The drawing under review shows one solid part. Ordinate dimensions are in mm from its lowest x, y, z. A direction names the side the tool comes from. Coordinates: 2 decimals unless noted, no trailing zeros. Write each loop counter-clockwise with the first axis right and the second up, starting at its lowest first coordinate (ties: lowest second). Pieces come first, ordered by that corner, then holes.
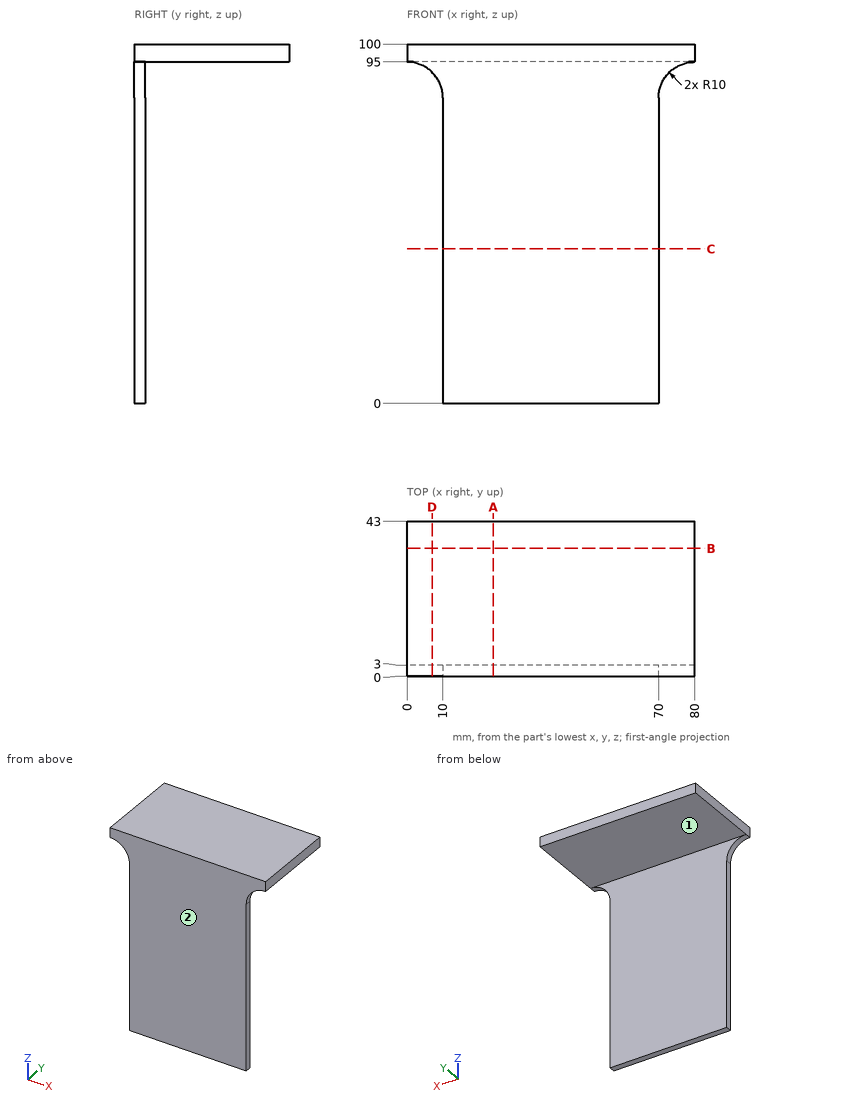
1) Consider section D-D (x = 7). Give the boundary of the cut face in (y, z), then the cut area to 3 significant figures.
2) Consider section A-A (x = 24). Give the boundary of the cut face in (y, z).
3) Clearance check with flat-ended pins moving along their axes: P1, Ø4, axis at x = 65.5, y = 6, coming from the -Z side; P2, Ø1.5, axis at y = 1, z = 62, coming from the -X side; P3, Ø12, axis at y = 12.5, z = 66, coming from the +X side; P4, Ø0.9, axis at y = 1, z = 55, coming from the +X side. State where each tip first meets the part, or that it passes through.
4) Consider section C-C (z = 43). Give the boundary of the cut face in (x, y).
5) Tool access review of the marked faces 1 and 2: name each direction out of +Z, -Z, +X, -X, +Y, -Y from which nothing blocks a thin tool from reaching the whole face with its end or side.
6) Consider section B-B (y = 35.5). Give the boundary of the cut face in (x, z).
7) For L1, parallel to Z at x = 53.5, y = 11.5; L2, parallel to Y at x = 23.5, z = 28, list the stretches that pass through material, from the lowest coordinate up.
Results:
1. outline: (0, 92.14) - (3, 92.14) - (3, 95) - (43, 95) - (43, 100) - (0, 100) - close
1. area: 224 mm2
2. outline: (0, 0) - (3, 0) - (3, 95) - (43, 95) - (43, 100) - (0, 100) - close
3. P1: stops at z = 95
3. P2: stops at x = 10
3. P3: passes through
3. P4: stops at x = 70
4. outline: (10, 0) - (70, 0) - (70, 3) - (10, 3) - close
5. face 1: -Z, +X, -X, +Y
5. face 2: +Z, -Z, +X, -X, -Y
6. outline: (0, 95) - (80, 95) - (80, 100) - (0, 100) - close
7. L1: z = 95 to 100
7. L2: y = 0 to 3
